The model under review builds one solid part; all positions refer to its coordinate system, in mm. Round coordinates to 2 decimals unless told otherwise and drop trailing zeros. Order: outer loops, then holes, each group sorted by start corner. A loop starts at its lowest first (then second) coordinate and runs counter-clockwise, first axis right, second up. Notation, with made-up numbers: M 2,53.25 L 52,53.25 A25 cw 52,68.25 Z; hole C 26,48 d2. An arc over 180 degrees is marked long. Use a Markdown table: item, result. Add a question column.
1. Consider section D-D on x = -21. State the section outline as (y, z) points.
2. Consider section B-B on x = 0.5. State the section outline as (y, z) points.
3. Consider section C-C on y = -12. State the section outline as (x, z) points, then the cut area to 3 significant figures.
4. To check wall thickness, follow probe 1 along Z at (x, y) = (-25, -44); probe 2 along X at (y, z) = (-77.5, 11); probe 3 along X at (y, z) = (-44, -60). State the ranges of each line that lie inside material, in increasing order.
5. Insertion check: P1, Ø8, axis at y = -48.5, z = -72, coming from the +X side; P2, Ø6, axis at y = -85, z = 40.5, coming from the -X side; P3, Ø10, axis at y = -46.5, z = 37.5, coming from the +X side. Each pin has a flat end and moves straight along its axis. Give the tip position at first contact, or say it passes through.
6. Consider section A-A on z = -8.5. State the section outline as (x, y) points, then the cut area to 3 significant figures.
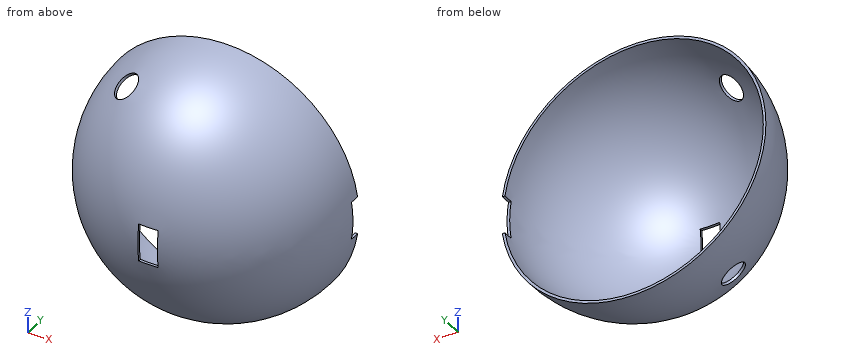
Autodesk Inventor part; units mm, degrees
ref_plane "Arbeitsebene1" through (0, -102, 0) normal (0, 1, 0) x (-1, 0, 0)
ref_plane "YZ Plane" through (0, 0, 0) normal (1, 0, 0) x (0, 1, 0)
ref_plane "XZ Plane" through (0, 0, 0) normal (0, 1, 0) x (-1, 0, 0)
sketch "Skizze2" plane through (0, 0, 0) normal (0, 0, 1) x (1, 0, 0)
  line L0 (100, 0) -> (102, 0)
  arc A0 (0, -102) -> (102, 0) centre (0, 0) ccw
  line L1 (0, -102) -> (0, -100)
  arc A1 (0, -100) -> (100, 0) centre (0, 0) ccw
  point P0 (0, 0)
  point P1 (0, -101)
  point P2 (101, 0)
  dimension "d0" = 2
  dimension "d1" = 2
  dimension "d3" = 100
  dimension "d4" = 100
revolve "Umdrehung1" add sketch "Skizze2" angle 360 about axis through (0, -102, 0) along (0, 1, 0)
ref_plane "Arbeitsebene1" through (0, -102, 0) normal (0, 1, 0) x (-1, 0, 0)
sketch "Skizze3" plane through (0, -102, 0) normal (0, 1, 0) x (-1, 0, 0)
  line L0 (7.5, 15) -> (-7.5, 15)
  line L1 (-7.5, 15) -> (-7.5, -15)
  line L2 (-7.5, -15) -> (7.5, -15)
  line L3 (7.5, -15) -> (7.5, 15)
  point P0 (0, 0)
  point P1 (7.5, 0)
  point P2 (0, 15)
  dimension "d6" = 15
  dimension "d7" = 30
extrude "Extrusion1" cut sketch "Skizze3" along normal through all both and the other way through all
sketch "Skizze4" plane through (0, 0, 0) normal (1, 0, 0) x (0, 1, 0)
  line L0 (7.5, 15) -> (-7.5, 15)
  line L1 (-7.5, 15) -> (-7.5, -15)
  line L2 (-7.5, -15) -> (7.5, -15)
  line L3 (7.5, -15) -> (7.5, 15)
  point P0 (0, 0)
  point P1 (0, 0)
  point P2 (7.5, 0)
  point P3 (0, 15)
  point P4 (-7.5, 0)
  dimension "d10" = 15
  dimension "d11" = 30
extrude "Extrusion2" cut sketch "Skizze4" along normal through all
sketch "Skizze6" plane through (0, 0, 0) normal (0, 1, 0) x (1, 0, 0)
  line L0 (0, 0) -> (-94.1178, 163.0168) construction
  line L1 (0, 0) -> (188.2356, 0) construction
  line L2 (0, 0) -> (-95.3588, -165.1662) construction
  line L3 (0, 0) -> (190.7175, 0) construction
  arc A0 (100.891, 15) -> (100.891, -15) centre (0, 0) ccw construction
  point P0 (-51, -88.3346)
  point P1 (-51, 88.3346)
  dimension "d16" = 120
  dimension "d17" = 120
ref_plane "Arbeitsebene7" through (-51, 0, -88.3346) normal (1, 0, 0) x (0, 1, 0)
sketch "Skizze14" plane through (-51, 0, -88.3346) normal (1, 0, 0) x (0, 1, 0)
  circle A0 centre (0, 88.3346) radius 88.3346 construction
  line L0 (0, 88.3346) -> (-48.5836, 172.4838) construction
  line L1 (0, 188.3346) -> (0, -11.6654) construction
  line L2 (0, 88.3346) -> (-62.5691, -20.0382) construction
  point P0 (0, 103.3346)
  point P1 (0, 73.3346)
  point P2 (-44.1673, 164.8346)
  point P3 (-44.1673, 11.8346)
  dimension "d38" = 176.6692
  dimension "d39" = 30
  dimension "d40" = 30
sketch "Skizze16" plane through (0, 0, 0) normal (0, 1, 0) x (1, 0, 0)
  circle A0 centre (0, 0) radius 102 construction
  arc A1 (100.891, 15) -> (100.891, -15) centre (0, 0) ccw construction
  arc A2 (100.6119, -15) -> (100.6119, 15) centre (0, 0) ccw construction
  point P0 (101.7239, 0)
  dimension "d37" = 204
ref_plane "Arbeitsebene8" through (-51, -44.1673, -76.5) normal (-0.5, -0.433, -0.75) x (0.6547, -0.7559, 0)
ref_plane "Arbeitsebene9" through (-51, -44.1673, 76.5) normal (-0.5, -0.433, 0.75) x (0.6547, -0.7559, 0)
sketch "Skizze17" plane through (-51, -44.1673, -76.5) normal (-0.5, -0.433, -0.75) x (0.6547, -0.7559, 0)
  point P0 (0, 0)
  point P1 (0, 0)
hole "Bohrung3" at (-51, -44.1673, -76.5) direction (0.5, 0.433, 0.75) diameter 21 depth 8 tip angle 118
sketch "Skizze18" plane through (-51, -44.1673, 76.5) normal (-0.5, -0.433, 0.75) x (0.6547, -0.7559, 0)
  point P0 (0, 0)
  point P1 (0, 0)
hole "Bohrung4" at (-51, -44.1673, 76.5) direction (0.5, 0.433, -0.75) diameter 21 depth 8 tip angle 118
properties part number "Schale_V1"
Answer block:
| question | item | result |
|---|---|---|
| 1 | outline | M 0,-99.81 L 0,-97.77 A97.77 cw 0,97.77 L 0,99.81 A99.81 ccw Z |
| 2 | outline | M -100.89,-15 A102 ccw 0,-102 L 0,-100 A100 cw -98.87,-15 Z; M -100.89,15 L -98.87,15 A100 cw 0,100 L 0,102 A102 ccw Z |
| 3 | outline | C 0,0 d202.58; hole C 0,0 d198.55 |
| 3 | area | 1,270 mm^2 |
| 4 | probe 1 | -88.56 to -86.25, 86.25 to 88.56 |
| 4 | probe 2 | -65.4 to -62.23, 62.23 to 65.4 |
| 4 | probe 3 | -69.77 to -66.81, 66.81 to 69.77 |
| 5 | P1 | x = 59.55 |
| 5 | P2 | x = -45.77 |
| 5 | P3 | x = 86.07 |
| 6 | outline | M -101.65,0 A101.65 ccw -7.5,-101.37 L -7.5,-99.36 A99.64 cw -99.64,0 Z; M 7.5,-101.37 A101.65 ccw 101.37,-7.5 L 99.36,-7.5 A99.64 cw 7.5,-99.36 Z |
| 6 | area | 589 mm^2 |
